```python
from build123d import *

# Parameters (mm, degrees)
F0_R     = 26.5
F1_DEPTH = 58
F3_DEPTH = 5


with BuildPart() as f1:
    # F0 (on Front) → F1 (new body)
    with BuildSketch(Plane.XZ):
        Polygon((3.743613, -39.952497), (27.196158, -10.655544), (13.550526, 24.303433), (-23.547653, 29.965456), (-47.000198, 0.668504), (-33.354566, -34.290473), align=None)
        with Locations((-9.90202, -4.99352)):
            Circle(F0_R, mode=Mode.SUBTRACT)
    extrude(amount=F1_DEPTH)

    # F2 (on face) → F3 (join)
    with BuildSketch(Plane(origin=(0, 0, 0), x_dir=(-1, 0, 0), z_dir=(0, 1, 0))):
        Polygon((23.547653, 29.965456), (-13.550526, 24.303433), (-27.196158, -10.655544), (-3.743613, -39.952497), (33.354566, -34.290473), (47.000198, 0.668504), align=None)
    extrude(amount=F3_DEPTH)


solid = f1.part
```
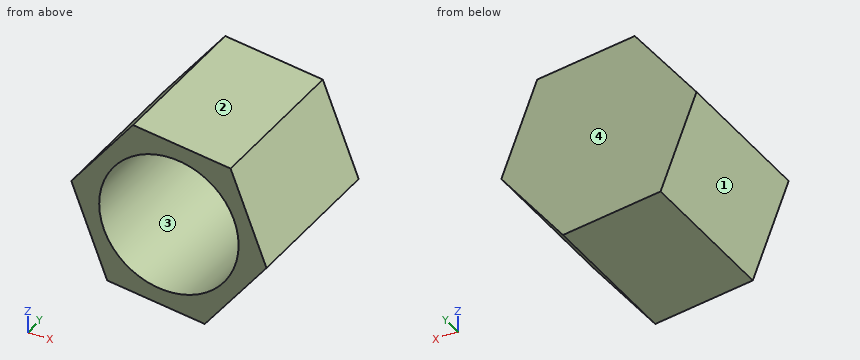
Geometry check sheet. Reference: the model listing, model coordinates, mm. Face numbers are marked on the shaded views. Coordinates: 2 decimals unless noted, no trailing zeros. Write each loop counter-clockwise with the first axis right and the second up, starting at its lowest first coordinate (ties: lowest second). Pieces come first, ordered by that corner, then holes. Notation, with made-up numbers: M 14.5,4.25 L 55.5,4.25 A26 ccw 55.5,30.25 Z; hole C 48,-16.5 d2. An arc over 180 degrees is marked long. One line per item, written item: value. Start each with the question number.
(1) Release check for a two-part mould opening along Z. For the marked faces 1, 2, 3 and 4 record: released by +Z, released by -Z, zero draft, split by the parting line, or undercut.
(2) Sectioned sample at B-B, the plane z = -1. Enter the section's corners in (x, y).
(3) Sectioned sample at D-D, the plane y = -26. Enter the section's corners in (x, z), and give its area (3 significant figures).
(4) Sectioned sample at C-C, the plane x = -15.5. Enter the section's corners in (y, z).
(5) Sectioned sample at A-A, the plane y = 1.5. Enter the section's corners in (x, z).
(6) Scan lines: line 1 along Y through (x, z) = (-16, -7.5); line 2 along Z through (x, y) = (-11, -19); line 3 along Z through (x, y) = (-2, -51). Record each from-to range of solid material in increasing order. Write a range as [from, to].
(7) Depth check by flat-ended pin: pin 1 (1 mm diameter, centred on x = 18.5, y = -48, fed in from -Z); pin 2 (4 mm diameter, centred on y = -16.5, z = -4.5, fed in from -X); pin 3 (4 mm diameter, centred on y = -10.5, z = -25, fed in from -X). Enter the tip coordinate at first touch or a pass-through.
Filled sheet:
1. face 1: released by -Z
1. face 2: released by +Z
1. face 3: undercut
1. face 4: zero draft
2. outline: M -46.35,-58 L -36.1,-58 L -36.1,0 L 16.3,0 L 16.3,-58 L 23.43,-58 L 23.43,5 L -46.35,5 Z
3. outline: M -47,0.67 L -33.35,-34.29 L 3.74,-39.95 L 27.2,-10.66 L 13.55,24.3 L -23.55,29.97 Z; hole C -9.9,-4.99 d53
3. area: 1,450 mm²
4. outline: M -58,-37.02 L 5,-37.02 L 5,28.74 L -58,28.74 L -58,20.91 L 0,20.91 L 0,-30.9 L -58,-30.9 Z
5. outline: M -47,0.67 L -33.35,-34.29 L 3.74,-39.95 L 27.2,-10.66 L 13.55,24.3 L -23.55,29.97 Z
6. line 1: [0, 5]
6. line 2: [-37.7, -31.47], [21.48, 28.05]
6. line 3: [-39.08, -30.29], [20.3, 26.68]
7. pin 1: z = -22.14
7. pin 2: x = -45.76
7. pin 3: x = -37.76
